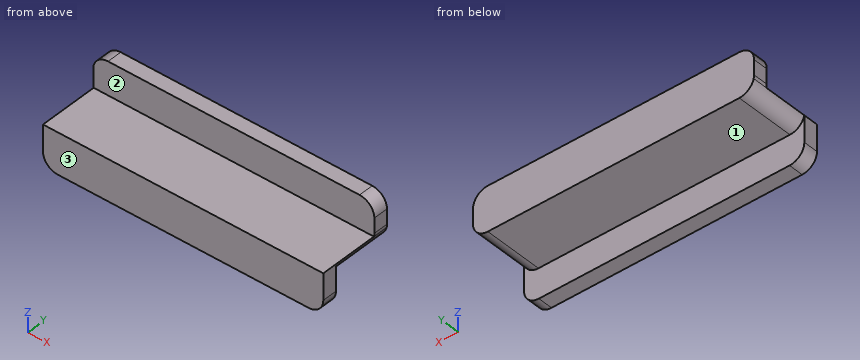
from build123d import *

# Parameters (mm, degrees)
BOSS_EXTRUDE1_DEPTH = 2
BOSS_EXTRUDE2_START = -10
BOSS_EXTRUDE2_DEPTH = 10
BOSS_EXTRUDE3_DEPTH = 2


with BuildPart() as part:
    # Sketch1 → Boss-Extrude1 (new body)
    with BuildSketch(Plane(origin=(0, 0, 0), x_dir=(1, 0, 0), z_dir=(0, 1, 0))):
        with BuildLine():
            Line((-17, -3), (17, -3))
            ThreePointArc((17, -3), (18.414213562, -2.414213562), (19, -1))
            Line((19, -1), (19, 1))
            ThreePointArc((19, 1), (18.414213562, 2.414213562), (17, 3))
            Line((17, 3), (-17, 3))
            ThreePointArc((-17, 3), (-18.414213562, 2.414213562), (-19, 1))
            Line((-19, 1), (-19, -1))
            ThreePointArc((-19, -1), (-18.414213562, -2.414213562), (-17, -3))
        make_face()
    extrude(amount=BOSS_EXTRUDE1_DEPTH)

    # Sketch2 → Boss-Extrude2 (add)
    with BuildSketch(Plane(origin=(0, 2, 0), x_dir=(1, 0, 0), z_dir=(0, 1, 0)).offset(BOSS_EXTRUDE2_START)):
        with BuildLine():
            Line((17, 3), (-17, 3))
            ThreePointArc((-17, 3), (-18.241842888, 2.567745592), (-18.946893714, 1.457826241))
            Line((-18.946893714, 1.457826241), (18.946893714, 1.457826241))
            ThreePointArc((18.946893714, 1.457826241), (18.241842888, 2.567745592), (17, 3))
        make_face()
    extrude(amount=BOSS_EXTRUDE2_DEPTH)

    # Sketch4 → Boss-Extrude3 (add)
    with BuildSketch(Plane.XZ.offset(8)):
        with BuildLine():
            Line((-18.946893714, -1.457826241), (-18.946893714, -5))
            ThreePointArc((-18.946893714, -5), (-18.361107276, -6.414213562), (-16.946893714, -7))
            Line((-16.946893714, -7), (16.946893714, -7))
            ThreePointArc((16.946893714, -7), (18.361107276, -6.414213562), (18.946893714, -5))
            Line((18.946893714, -5), (18.946893714, -1.457826241))
            ThreePointArc((18.946893714, -1.457826241), (18.241842888, -2.567745592), (17, -3))
            Line((17, -3), (-17, -3))
            ThreePointArc((-17, -3), (-18.241842888, -2.567745592), (-18.946893714, -1.457826241))
        make_face()
    extrude(amount=-BOSS_EXTRUDE3_DEPTH)


solid = part.part
Check sheet for the modelled part. Datum: model origin and axes. Units: mm. Face numbers are marked on the shaded views. A direction names the side the tool comes from. Round coordinates to 2 decimals unless told otherwise and drop trailing zeros. Order: outer loops, then holes, each group sorted by start corner. A loop starts at its lowest first (then second) coordinate and runs counter-clockwise, first axis right, second up.
Q1. Cross-section at C-C, the plane z = -2.5. Enter the section's corners in (x, y), plus the area to 3 significant figures.
Filled sheet:
outline: (-18.95, -8) - (18.95, -8) - (18.95, -6) - (18.32, -6) - (18.32, 2) - (-18.32, 2) - (-18.32, -6) - (-18.95, -6) - close
area: 369 mm2
Q2. Cross-section at B-B, the plane y = 0.5. Enter the section's corners in (x, z).
Filled sheet:
outline: (-19, -1) arc R2 ccw to (-17, -3) - (17, -3) arc R2 ccw to (19, -1) - (19, 1) arc R2 ccw to (17, 3) - (-17, 3) arc R2 ccw to (-19, 1) - close
Q3. Depth check by flat-ended pin: P1, Ø1, axis at y = -6.5, z = -3.5, coming from the +X side; P2, Ø5, axis at x = -0.5, y = -3, coming from the -Z side; P3, Ø2, axis at x = -1, z = 1, coming from the -Y side; P4, Ø3, axis at y = -1.5, z = -6, coming from the +X side. Enter the tip coordinate at first touch or a pass-through.
Filled sheet:
P1: stops at x = 18.95
P2: stops at z = -3
P3: stops at y = 0
P4: passes through
Q4. Cross-section at A-A, the plane x = -0.5. Enter the section's corners in (y, z), plus the area to 3 significant figures.
Filled sheet:
outline: (-8, -7) - (-6, -7) - (-6, -3) - (2, -3) - (2, 3) - (0, 3) - (0, -1.46) - (-8, -1.46) - close
area: 32.3 mm2
Q5. Set-up check for the marked faces 1, 2 and 3: record each of +Z, -Z, +X, -X, +Y, -Y from which the full face is reachable in a straight line by a thin tool's end or side.
Filled sheet:
face 1: -Z, +X, -X, +Y
face 2: +Z, +X, -X, -Y
face 3: +Z, -Z, +X, -X, -Y
Q6. Scan lines: L1, parallel to X at y = -6.75, z = -2; L2, parallel to Z at x = -5, y = -3.25; L3, parallel to Y at x = 12.5, z = 1.5. Record each from-to range of solid material in increasing order.
Filled sheet:
L1: x = -18.95 to 18.95
L2: z = -3 to -1.46
L3: y = 0 to 2
Q7. Cross-section at D-D, the plane y = -7. Enter the section's corners in (x, z).
Filled sheet:
outline: (-18.95, -5) arc R2 ccw to (-16.95, -7) - (16.95, -7) arc R2 ccw to (18.95, -5) - (18.95, -1.46) - (-18.95, -1.46) - close
